Geometry check sheet. Reference: drawing and pictorial views, mm from the part's lowest x, y, z. A direction names the side the tool comes from. Give positions to 0.01 mm unless a question says otherwise; leave off trailing zeros. Order: outer loops, then holes, each group sorted by start corner. A loop starts at its lowest first (then second) coordinate and runs counter-clockwise, first axis right, second up.
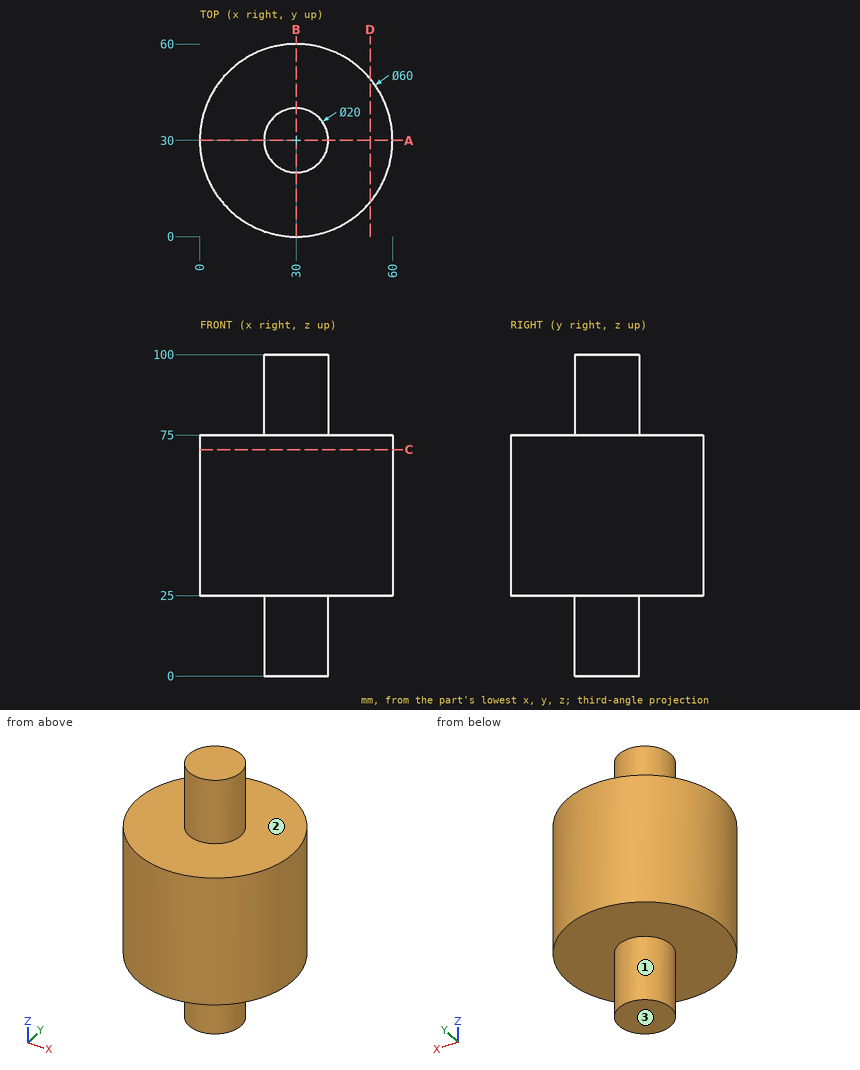
(1) Gauge pin test, flat ends, axial feed: pin 1 Ø1 at (x, z) = (26.5, 78.5) entering from +Y; pin 2 Ø4 at (x, y) = (8, 45) entering from +Z; pin 3 Ø18 at (x, y) = (16, 25) entering from -Z; pin 4 Ø5 at (y, z) = (30, 80.5) entering from -X. Record the tip position at first contact, or that the pin passes through.
Response values:
pin 1: stops at y = 39.54
pin 2: stops at z = 75
pin 3: stops at z = 0
pin 4: stops at x = 20
(2) Cross-section at D-D on x = 53. Enter the section's corners in (y, z), then the cut area to 3 significant figures.
Response values:
outline: (10.74, 25) - (49.26, 25) - (49.26, 75) - (10.74, 75) - close
area: 1,930 mm2
(3) Material ranges on L1, parallel to Z at x = 47.5, y = 13; L2, parallel to X at y = 21, z = 83.5; L3, parallel to X at y = 38, z = 56, recorded low to high.
Response values:
L1: z = 25 to 75
L2: x = 25.64 to 34.36
L3: x = 1.09 to 58.91
(4) Set-up check for the marked faces 1, 2 and 3: record each of +Z, -Z, +X, -X, +Y, -Y from which the full face is reachable in a straight line by a thin tool's end or side.
Response values:
face 1: -Z
face 2: +Z
face 3: -Z, +X, -X, +Y, -Y
(5) Cross-section at A-A on y = 30. Enter the section's corners in (x, z).
Response values:
outline: (0, 25) - (20, 25) - (20, 0) - (40, 0) - (40, 25) - (60, 25) - (60, 75) - (40, 75) - (40, 100) - (20, 100) - (20, 75) - (0, 75) - close
(6) Cross-section at C-C on z = 70.5. Enter the section's corners in (x, y).
Response values:
outline: circle Ø60 at (30, 30)
